The model under review builds one solid part; all positions refer to its coordinate system, in mm. Face numbers are marked on the shaded views. A direction names the side the tool comes from. Coordinates: 2 decimals unless noted, no trailing zeros. Order: outer loops, then holes, each group sorted by start corner. A loop starts at its lowest first (then second) coordinate and runs counter-clockwise, first axis right, second up. Notation, with made-up numbers: (75, 44.25) - (105, 44.25) arc R21 ccw to (105, 63.25) - close; hole circle Ø9 at (-36, -14). An arc over 180 degrees is marked (long way). Answer in a Markdown table with one row per item.
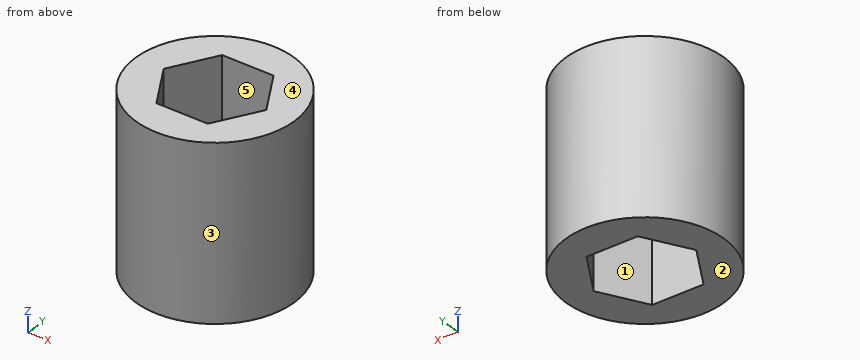
Autodesk Inventor part; units mm, degrees
ref_plane "YZ Plane" through (0, 0, 0) normal (1, 0, 0) x (0, 1, 0)
ref_plane "XZ Plane" through (0, 0, 0) normal (0, 1, 0) x (-1, 0, 0)
ref_plane "XY Plane" through (0, 0, 0) normal (0, 0, 1) x (1, 0, 0)
sketch "Sketch1" plane through (0, 0, 0) normal (0, 0, 1) x (1, 0, 0)
  line L0 (2.7496, 4.7625) -> (5.4993, 0)
  line L1 (5.4993, 0) -> (2.7496, -4.7625)
  line L2 (2.7496, -4.7625) -> (-2.7496, -4.7625)
  line L3 (-2.7496, -4.7625) -> (-5.4993, 0)
  line L4 (-5.4993, 0) -> (-2.7496, 4.7625)
  line L5 (-2.7496, 4.7625) -> (2.7496, 4.7625)
  circle A0 centre (0, 0) radius 8.7313
  circle A1 centre (0, 0) radius 5.4993 construction
  dimension "d0" = 9.525
  dimension "d2" = 17.4625
  dimension "d3" = 3.232
extrude "Extrusion1" add sketch "Sketch1" against normal blind 19.05
thicken "Thicken Hex" operation add thickness 0.127 both sides no extend neighbours yes toward (-0.8660254, 0.5, 0) faces at (-4.5827, 1.5875, -6.35) (-3.6662, -3.175, -6.35) (0.9165, -4.7625, -6.35) (-0.9165, 4.7625, -6.35) (3.6662, 3.175, -6.35) (4.5827, -1.5875, -6.35)
equation "\"d0\" = hexSize"
equation "\"d2\" = exteriorDiameter"
equation "\"d4\" = length"
equation "\"d6\" = printSpacing"
equation "\"d7\" = printSpacing"
equation "\"hexSize\" = 9.525"
equation "\"exteriorDiameter\" = 17.4625"
equation "\"length\" = 19.05"
equation "\"printSpacing\" = 0.127"
properties part number "3_8x11_16x3_4-hexBearing" material "PC/ABS Plastic"
Item 1: Mouldability with a two-part tool opening along X and no side actions: class the marked faces 1, 2 and 3 as +X half, -X half, draft (parallel to the pull), parting line (faces both ways), or undercut.
Check values:
| item | result |
|---|---|
| face 1 | undercut |
| face 2 | draft |
| face 3 | parting line |
Item 2: To check wall thickness, follow line 1 (Y direction, x = -1.75, z = -18); line 2 (Y direction, x = -5, z = -10.75); line 3 (X direction, y = 2, z = -5.5). State the ranges of each line that lie inside material, in increasing order. Write a range as from..to.
Check values:
| item | result |
|---|---|
| line 1 | -8.55..-4.89, 4.89..8.55 |
| line 2 | -7.16..-1.12, 1.12..7.16 |
| line 3 | -8.5..-4.49, 4.49..8.5 |
Item 3: Tool access review of the marked faces 4 and 5: name each direction out of +Z, -Z, +X, -X, +Y, -Y from which nothing blocks a thin tool from reaching the whole face with its end or side.
Check values:
| item | result |
|---|---|
| face 4 | +Z, +X, -X, +Y, -Y |
| face 5 | +Z, -Z |
Item 4: Clearance check with flat-ended pins moving along their axes: pin 1 Ø5 at (y, z) = (-4, -8.5) entering from +X; pin 2 Ø1 at (x, z) = (-6, -6) entering from -Y; pin 3 Ø5 at (y, z) = (3, -3) entering from +X. State where each tip first meets the part, or that it passes through.
Check values:
| item | result |
|---|---|
| pin 1 | x = 8.6 |
| pin 2 | y = -6.78 |
| pin 3 | x = 8.72 |
Item 5: We need section C-C, the plane y = -1.5. Write out the cut boundary in (x, z).
Check values:
| item | result |
|---|---|
| outline | (-8.6, -19.05) - (-4.78, -19.05) - (-4.78, 0) - (-8.6, 0) - close; (4.78, -19.05) - (8.6, -19.05) - (8.6, 0) - (4.78, 0) - close |
Item 6: We need section A-A, the plane x = 0. Write out the cut boundary in (y, z).
Check values:
| item | result |
|---|---|
| outline | (-8.73, -19.05) - (-4.89, -19.05) - (-4.89, 0) - (-8.73, 0) - close; (4.89, -19.05) - (8.73, -19.05) - (8.73, 0) - (4.89, 0) - close |
Item 7: We need section D-D, the plane x = -7.5. Write out the cut boundary in (y, z).
Check values:
| item | result |
|---|---|
| outline | (-4.47, -19.05) - (4.47, -19.05) - (4.47, 0) - (-4.47, 0) - close |
Item 8: We need section B-B, the plane z = -5. Write out the cut boundary in (x, y).
Check values:
| item | result |
|---|---|
| outline | circle Ø17.46 at (0, 0); hole (-5.65, 0) - (-2.82, -4.89) - (2.82, -4.89) - (5.65, 0) - (2.82, 4.89) - (-2.82, 4.89) - close |
